Part model, mm, in its own coordinate system. A direction names the side the tool comes from. Coordinates: 2 decimals unless noted, no trailing zeros. Loops run counter-clockwise (first coordinate to the right, second up) from the corner with the lowest first, then second, coordinate; pieces in that order, holes last. Notation, with made-up numbers: (58.25, 4.5) -> (74.25, 4.5) arc R11 ccw to (74.25, 18.5) -> close; hole circle Ø8 at (33.25, -1). An arc over 180 degrees is marked (long way). Use one line per item in the form item = value. Start each with the question number.
(1) 3-axis set-ups, long thin cutter, end or side, ignore diameter. For faces 1 (the cylindrical face through (-9.139, 14.334, -15.135)), 2 (the cylindrical face through (-14.6, -11.2, 13.1)), 3 (the cylindrical face through (-8.08, 11.96, 24.04)): which of +Z, -Z, +X, -X, +Y, -Y reach the whole face in a straight line?
(2) Drill centre lines: L1, parallel to Z at x = -13.5, y = -11; L2, parallel to Z at x = -1.5, y = 10.5; L3, parallel to Y at x = -15.5, z = 23.3. Where is each one in solid material? Low to high. Write a range as [from, to].
(3) Mould opens along X. For faces 4 (the flat face through (-8, 13, 21.5)), 5 (the flat face through (5.4, -16.3, 0)), 6 (the cylindrical face through (-6, -7, 29)) say: +X half, -X half, draft (parallel to the pull), parting line (faces both ways), or undercut.
(4) Pin check, flat tips, straight feed: P1, Ø12, axis at y = 7, z = 10, coming from the -X side; P2, Ø3.5, axis at x = 8, y = -13.5, coming from the +Z side; P3, Ø3, axis at y = -14, z = 21.5, coming from the -X side. Stop position of each tip, or through.
(5) Band-saw the part on A-A on x = 0. Give the cut face in (y, z).
(6) Band-saw the part on B-B on y = 0. Give the cut face in (x, z).
(7) Band-saw the part on D-D on y = 4. Give the cut face in (x, z), then the cut area to 3 significant figures.
(8) Band-saw the part on C-C on z = 5.5. Give the cut face in (x, y).
```python
from build123d import *

# Parameters (mm, degrees)
CROQUIS1_R              = 18.4
SALIENTE_EXTRUIR1_DEPTH = 26.5
CROQUIS2_R              = 17
SALIENTE_EXTRUIR2_DEPTH = 30.7
CROQUIS3_R              = 1.5
CORTAR_EXTRUIR1_DEPTH   = 5
CROQUIS4_R              = 6
SALIENTE_EXTRUIR3_DEPTH = 6
CROQUIS5_R              = 3
SALIENTE_EXTRUIR4_DEPTH = 16


with BuildPart() as part:
    # Croquis1 → Saliente-Extruir1 (new body)
    with BuildSketch(Plane.XY):
        Circle(CROQUIS1_R)
    extrude(amount=SALIENTE_EXTRUIR1_DEPTH)

    # Croquis2 → Saliente-Extruir2 (add)
    with BuildSketch(Plane(origin=(0, 0, 0), x_dir=(-1, 0, 0), z_dir=(0, 0, -1))):
        Circle(CROQUIS2_R)
    extrude(amount=SALIENTE_EXTRUIR2_DEPTH)

    # Croquis3 → Cortar-Extruir1 (cut)
    with BuildSketch(Plane.XY.offset(26.5)):
        with Locations((-15.5, 0)):
            Circle(CROQUIS3_R)
        with Locations((-7.75, 13.423393759)):
            Circle(CROQUIS3_R)
        with Locations((7.75, 13.423393759)):
            Circle(CROQUIS3_R)
        with Locations((15.5, 0)):
            Circle(CROQUIS3_R)
        with Locations((7.75, -13.423393759)):
            Circle(CROQUIS3_R)
        with Locations((-7.75, -13.423393759)):
            Circle(CROQUIS3_R)
    extrude(amount=-CORTAR_EXTRUIR1_DEPTH, mode=Mode.SUBTRACT)

    # Croquis4 → Saliente-Extruir3 (add)
    with BuildSketch(Plane.XY.offset(26.5)):
        with Locations((0, -7)):
            Circle(CROQUIS4_R)
    extrude(amount=SALIENTE_EXTRUIR3_DEPTH)

    # Croquis5 → Saliente-Extruir4 (add)
    with BuildSketch(Plane.XY.offset(32.5)):
        with Locations((0, -7)):
            Circle(CROQUIS5_R)
    extrude(amount=SALIENTE_EXTRUIR4_DEPTH)


solid = part.part
```
A:
q1.face_1 = -Z
q1.face_2 = +Z, -Z
q1.face_3 = +Z
q2.L1 = [0, 26.5]
q2.L2 = [-30.7, 26.5]
q2.L3 = [-9.92, -1.5], [1.5, 9.92]
q3.face_4 = undercut
q3.face_5 = draft
q3.face_6 = parting line
q4.P1 = -18.37
q4.P2 = 26.5
q4.P3 = -13.5
q5.outline = (-18.4, 0) -> (-17, 0) -> (-17, -30.7) -> (17, -30.7) -> (17, 0) -> (18.4, 0) -> (18.4, 26.5) -> (-1, 26.5) -> (-1, 32.5) -> (-4, 32.5) -> (-4, 48.5) -> (-10, 48.5) -> (-10, 32.5) -> (-13, 32.5) -> (-13, 26.5) -> (-18.4, 26.5) -> close
q6.outline = (-18.4, 0) -> (-17, 0) -> (-17, -30.7) -> (17, -30.7) -> (17, 0) -> (18.4, 0) -> (18.4, 26.5) -> (17, 26.5) -> (17, 21.5) -> (14, 21.5) -> (14, 26.5) -> (-14, 26.5) -> (-14, 21.5) -> (-17, 21.5) -> (-17, 26.5) -> (-18.4, 26.5) -> close
q7.outline = (-17.96, 0) -> (-16.52, 0) -> (-16.52, -30.7) -> (16.52, -30.7) -> (16.52, 0) -> (17.96, 0) -> (17.96, 26.5) -> (-17.96, 26.5) -> close
q7.area = 1,970 mm²
q8.outline = circle Ø36.8 at (0, 0)
